from build123d import *

# Parameters (mm, degrees)
PAD_DEPTH = 3.25


with BuildPart() as pad:
    # Sketch001 → Pad (new body, symmetric)
    with BuildSketch(Plane.YZ):
        with BuildLine():
            Line((8.5, 0), (8.5, 17))
            Line((8.5, 17), (14, 17))
            Line((14, 17), (18.511951, 29.405352))
            ThreePointArc((32.805084, 20.799482), (30.884444, 33.78194), (18.511951, 29.405352))
            Line((14, 0), (32.805084, 20.799482))
            Line((8.5, 0), (14, 0))
        make_face()
        with BuildLine():
            Line((-32.80508, 20.799452), (-13.999963, 0))
            Line((-13.999963, 0), (-8.499963, 0))
            Line((-8.499963, 0), (-8.499963, 17))
            Line((-8.499963, 17), (-13.999963, 17))
            Line((-13.999963, 17), (-18.511955, 29.405337))
            ThreePointArc((-18.511955, 29.405337), (-30.884451, 33.781911), (-32.80508, 20.799452))
        make_face()
    extrude(amount=PAD_DEPTH, both=True)


with BuildPart() as obj1:
    # Sketch → Revolution (revolve)
    with BuildSketch(Plane.YZ):
        Polygon((8, 0), (6.92, 0.623538), (6.92, 16.376462), (8, 17), (12, 17), (13, 0), align=None)
    revolve(axis=Axis((0, 0, 0), (0, 0, 1)))

    # Fusion: union Pad
    add(pad.part)


solid = obj1.part
Build history of the part. All positions in model axes, mm. A direction names the side the tool comes from. Round coordinates to 2 decimals unless told otherwise and drop trailing zeros. Loops run counter-clockwise (first coordinate to the right, second up) from the corner with the lowest first, then second, coordinate; pieces in that order, holes last. Notation, with made-up numbers: (63.25, -19) -> (85.25, -19) arc R7 ccw to (85.25, -12) -> close; hole circle Ø4 at (-22, 28.25). An arc over 180 degrees is marked (long way). Answer in a Markdown table with one row per item.
Item 1: Saw through at D-D (z = 11.5). Write the cut outline in (x, y), and give its area (3 significant figures).
Answers below:
| item | result |
|---|---|
| outline | (-3.25, -24.4) -> (3.25, -24.4) -> (3.25, -11.89) arc R12.32 ccw to (3.25, 11.89) -> (3.25, 24.4) -> (-3.25, 24.4) -> (-3.25, 11.89) arc R12.32 ccw to (-3.25, -11.89) -> close; hole circle Ø13.84 at (0, 0) |
| area | 486 mm² |
Item 2: Mould opens along Y. For faces 1 (the flat face through (0.046, -16.224, 23.116)), 2 (the flat face through (6, 6, 0)), 3 (the flat face through (0.046, -23.534, 10.545)) say: +Y half, -Y half, draft (parallel to the pull), parting line (faces both ways), or undercut.
Answers below:
| item | result |
|---|---|
| face 1 | undercut |
| face 2 | draft |
| face 3 | -Y half |
Item 3: Saw through at C-C (z = 22). Write the cut outline in (x, y), and give its area (3 significant figures).
Answers below:
| item | result |
|---|---|
| outline | (-3.25, -33.71) -> (3.25, -33.71) -> (3.25, -15.82) -> (-3.25, -15.82) -> close; (-3.25, 15.82) -> (3.25, 15.82) -> (3.25, 33.71) -> (-3.25, 33.71) -> close |
| area | 233 mm² |
Item 4: Pin check, flat tips, straight feed: pin 1 (12 mm diameter, centred on x = -6, y = 5.5, fed in from -Z); pin 2 (7 mm diameter, centred on y = -24.5, z = 20.5, fed in from +X); pin 3 (4 mm diameter, centred on y = -26.5, z = 29.5, fed in from -X); pin 4 (1.5 mm diameter, centred on x = 3, z = 29.5, fed in from -Y). Stop position of each tip, or through.
Answers below:
| item | result |
|---|---|
| pin 1 | stops at z = 0 |
| pin 2 | stops at x = 3.25 |
| pin 3 | stops at x = -3.25 |
| pin 4 | stops at y = -34.7 |
Item 5: Saw through at A-A (x = 0). Write the cut outline in (y, z), and give its area (3 significant figures).
Answers below:
| item | result |
|---|---|
| outline | (-32.81, 20.8) -> (-14, 0) -> (-8, 0) -> (-6.92, 0.62) -> (-6.92, 16.38) -> (-8, 17) -> (-14, 17) -> (-18.51, 29.41) arc R8.5 ccw (long way) to start; (6.92, 0.62) -> (8, 0) -> (14, 0) -> (32.81, 20.8) arc R8.5 ccw (long way) to (18.51, 29.41) -> (14, 17) -> (8, 17) -> (6.92, 16.38) -> close |
| area | 1,060 mm² |
Item 6: Drill centre lines: L1, parallel to Y at x = 0, z = 5; L2, parallel to X at y = 0, z = 8.75; L3, parallel to Y at x = 2.25, z = 7.5. Where is each one in solid material? Low to high. Write a range as [from, to].
Answers below:
| item | result |
|---|---|
| L1 | y = [-18.52, -6.92], [6.92, 18.52] |
| L2 | x = [-12.49, -6.92], [6.92, 12.49] |
| L3 | y = [-20.78, -6.54], [6.54, 20.78] |
Item 7: Saw through at B-B (y = 0). Write the cut outline in (x, z).
Answers below:
| item | result |
|---|---|
| outline | (-13, 0) -> (-8, 0) -> (-6.92, 0.62) -> (-6.92, 16.38) -> (-8, 17) -> (-12, 17) -> close; (6.92, 0.62) -> (8, 0) -> (13, 0) -> (12, 17) -> (8, 17) -> (6.92, 16.38) -> close |
Item 8: Which spindle directions (+Z, -Z, +X, -X, +Y, -Y) get a long thin tool onto all of the face, cutting with end or side? Do faces 4 (the flat face through (-8.2, -0.2, 17)), 5 (the cylindrical face through (0.05, -30.7, 33.89)). Say none if no direction does.
Answers below:
| item | result |
|---|---|
| face 4 | +Z, +X, -X |
| face 5 | +X, -X |
